Model file for the job. Use its own axes, mm. A direction names the side the tool comes from. Round coordinates to 2 decimals unless told otherwise and drop trailing zeros. Order: outer loops, then holes, each group sorted by start corner. A loop starts at its lowest first (then second) coordinate and runs counter-clockwise, first axis right, second up. Notation, with made-up numbers: (33, -4.75) -> (79, -4.75) arc R25 ccw to (79, 9.25) -> close; hole circle Ø7 at (49, 83). An arc over 180 degrees is marked (long way). Answer as CSV lines item,"result".
```python
from build123d import *

# Parameters (mm, degrees)
F0_W      = 23.49
F0_H      = 117.79
F1_DEPTH  = 6.7
F2_T      = -2.5
F1_FACE_W = 23.49
F1_FACE_H = 6.7
F3_DEPTH  = 3


with BuildPart() as f1:
    # F0 (on Front) → F1 (new body)
    with BuildSketch(Plane.XZ):
        Rectangle(F0_W, F0_H)
    extrude(amount=-F1_DEPTH)

    # F2
    f2_openings = [f1.faces().sort_by_distance(p)[0] for p in [
        (0, 0, 0),
    ]]
    offset(amount=F2_T, openings=f2_openings)

    # F1_face (on face) → F3 (cut)
    with BuildSketch(Plane(origin=(0, 3.35, -58.895), x_dir=(1, 0, 0), z_dir=(0, 0, -1))):
        Rectangle(F1_FACE_W, F1_FACE_H)
    extrude(amount=-F3_DEPTH, mode=Mode.SUBTRACT)


solid = f1.part
```
Q1. Wall check: L1, parallel to X at y = 4, z = 24 (3 decimals); L2, parallel to Y at x = -5.5, z = -40; L3, parallel to Z at x = -0.75, y = 2.5 (3 decimals). Give the ranges that are in metal, low to high. Write a range as [from, to].
Checks:
L1,"[-11.745, -9.245], [9.245, 11.745]"
L2,"[4.2, 6.7]"
L3,"[56.395, 58.895]"
Q2. Saw through at C-C (z = 18.5). Write the cut outline in (x, y) (3 decimals), plus the area to 3 significant figures.
Checks:
outline,"(-11.745, 0) -> (-9.245, 0) -> (-9.245, 4.2) -> (9.245, 4.2) -> (9.245, 0) -> (11.745, 0) -> (11.745, 6.7) -> (-11.745, 6.7) -> close"
area,"79.7 mm²"
Q3. Flat gauge pins, fed straight in: pin 1 (5.5 mm diameter, centred on x = -1, z = 27.5, fed in from -Y); pin 2 (3.5 mm diameter, centred on x = -4, y = 1.5, fed in from -Z) (3 decimals). Where does each tip first touch, or does it go through?
Checks:
pin 1,"y = 4.2"
pin 2,"z = 56.395"
Q4. Tool access for faces 4 (the flat face through (9.245, 2, -1)), 5 (the flat face through (-10, 0, 10)): list every direction of +Z, -Z, +X, -X, +Y, -Y with a clear straight run to the whole face (end or side of a thin tool).
Checks:
face 4,"-Z, -Y"
face 5,"+Z, -Z, +X, -X, -Y"
Q5. Mould opens along X. For faces 1 (the flat face through (0, 4.2, 1)), 2 (the flat face through (-11.745, 3, 1)), 3 (the flat face through (0, 3, 58.895)) say: +X half, -X half, draft (parallel to the pull), parting line (faces both ways), or undercut.
Checks:
face 1,"undercut"
face 2,"-X half"
face 3,"draft"
Q6. Saw through at B-B (x = 3). Write the cut outline in (y, z) (3 decimals), plus the area to 3 significant figures.
Checks:
outline,"(0, 56.395) -> (4.2, 56.395) -> (4.2, -55.895) -> (6.7, -55.895) -> (6.7, 58.895) -> (0, 58.895) -> close"
area,"297 mm²"
Q7. Saw through at A-A (y = 3). Write the cut outline in (x, z) (3 decimals), plus the area to 3 significant figures.
Checks:
outline,"(-11.745, -55.895) -> (-9.245, -55.895) -> (-9.245, 56.395) -> (9.245, 56.395) -> (9.245, -55.895) -> (11.745, -55.895) -> (11.745, 58.895) -> (-11.745, 58.895) -> close"
area,"620 mm²"
